Here's the drawing with two shaded views (mm, measured from the low corner). I have some questions. Round coordinates to 2 decimals unless told otherwise and drop trailing zeros. Loops run counter-clockwise (first coordinate to the right, second up) from the corner with the lowest first, then second, coordinate; pieces in that order, holes last. Notation, with made-up numbers: M 5.25,-31 L 12.25,-31 A17 cw 12.25,-18 Z; hole C -29,5 d11. An arc over 180 degrees is marked long. One line per item, written item: value. Start each with the question number.
Q1. I'm going to push a flat-ended pin straight in: pin 1 Ø1 at (x, z) = (2.5, 1.5) entering from -Y. Where does the tip first touch, or does it pass through?
Q2. Thinking about a two-plate mould opening in X: for the marked faces 1, 2 and 3, which applies, released by +X, released by -X, zero draft, split by the parting line, or undercut?
Q3. Imagine slicing it at C-C (z = 2.6). Please give me the cut outline in (x, y).
Q4. Imagine slicing it at A-A (x = 6.75). Please give me the cut outline in (y, z).
Q5. Please list where these lines run through material, in increasing order: line 1 along X through (y, z) = (5.25, 0.5) (1 decimal); line 2 along X through (y, z) = (7.25, 0.7); line 3 along Y through (x, z) = (5.75, 1.7).
Q6. Imagine slicing it at B-B (y = 5). Please give me the cut outline in (x, z).
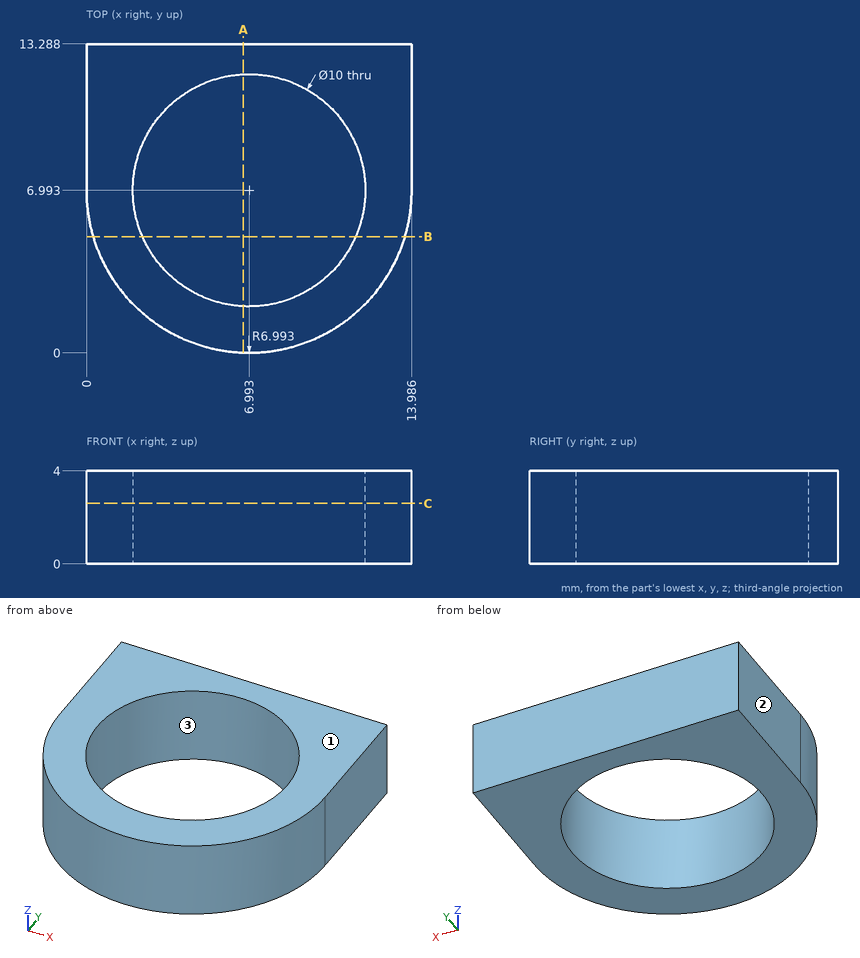
Report:
1. pin 1: stops at y = 1.25
2. face 1: zero draft
2. face 2: released by -X
2. face 3: undercut
3. outline: M 0,6.99 A6.99 ccw 13.99,6.99 L 13.99,13.29 L 0,13.29 Z; hole C 6.99,6.99 d10
4. outline: M 0,0 L 2,0 L 2,4 L 0,4 Z; M 11.99,0 L 13.29,0 L 13.29,4 L 11.99,4 Z
5. line 1: x = 0.2 to 2.3, 11.7 to 13.8
5. line 2: x = 0 to 2, 11.99 to 13.99
5. line 3: y = 0.11 to 2.15, 11.84 to 13.29
6. outline: M 0.29,0 L 2.41,0 L 2.41,4 L 0.29,4 Z; M 11.58,0 L 13.7,0 L 13.7,4 L 11.58,4 Z
